Source: CAD feature listing. Evaluate the final solid. Frame: model axes, mm. A direction names the side the tool comes from. Round coordinates to 2 decimals unless told otherwise and drop trailing zeros. Write each loop counter-clockwise with the first axis right and the second up, starting at its lowest first coordinate (ties: lowest second). Pieces come first, ordered by that corner, then holes.
```python
from build123d import *

# Parameters (mm, degrees)
F0_R       = 13.85
F1_DEPTH   = 18.5
F2_R       = 1.5
F3_DEPTH   = 1
F4_R       = 2.5
F5_DEPTH   = 12.5
F6_SIZE2   = 3.4641016151
F6_SIZE    = 2
F6_2_SIZE2 = 3.4641016151
F6_2_SIZE  = 2
F8_D       = 2.5
F8_DEPTH   = 13.5
F8_TIP     = 0.7510757738


with BuildPart() as f1:
    # F0 (on Top) → F1 (new body)
    with BuildSketch(Plane.XY):
        Circle(F0_R)
    extrude(amount=F1_DEPTH)

    # F2 (on face) → F3 (join)
    with BuildSketch(Plane(origin=(0, 0, 0), x_dir=(1, 0, 0), z_dir=(0, 0, -1))):
        Circle(F2_R)
    extrude(amount=F3_DEPTH)

    # F4 (on face) → F5 (join)
    with BuildSketch(Plane.XY.offset(18.5)):
        Circle(F4_R)
    extrude(amount=F5_DEPTH)

    # F6
    f6_edges = [f1.edges().sort_by_distance(p)[0] for p in [
        (-13.85, 0, 18.5),
    ]]
    f6_side = f1.faces().sort_by_distance((-13.458263, 0, 18.5))[0]
    chamfer(f6_edges, length=F6_SIZE, length2=F6_SIZE2, reference=f6_side)

    # F6#2
    f6_2_edges = [f1.edges().sort_by_distance(p)[0] for p in [
        (-13.85, 0, 0),
    ]]
    f6_2_side = f1.faces().sort_by_distance((-13.458263, 0, 0))[0]
    chamfer(f6_2_edges, length=F6_2_SIZE, length2=F6_2_SIZE2, reference=f6_2_side)

    # F8
    with Locations(Plane(origin=(0, 0, 0), x_dir=(1, 0, 0), z_dir=(0, 0, -1))):
        with Locations((-9.5, 0), (0, 8), (9.5, 0), (0, -8)):
            Hole(F8_D / 2, depth=F8_DEPTH)
            with Locations((0, 0, -(F8_DEPTH + F8_TIP / 2))):  # 118° drill point
                Cone(0, F8_D / 2, F8_TIP, mode=Mode.SUBTRACT)


solid = f1.part
```
Q1. Line query: line 1 (Y direction, x = 0.25, z = 3); line 2 (Z direction, x = -2.25, y = -9.25); line 3 (Z direction, x = 0, y = 8). Output: solid intervals per line, ascending.
Q2. Pin query (flat end, axial travel): P1, Ø2, axis at x = 0, y = 8, coming from the +Z side; P2, Ø3, axis at x = 3.5, y = 0, coming from the -Z side; P3, Ø12, axis at x = 5.5, y = -2, coming from the +Z side; P4, Ø5, axis at y = -4.5, z = 25.5, coming from the +X side. Return the tip coordinate at first contact, or that it passes through.
Q3. Set-up query: faces 5 (the face through (-0.54, -2.44, 24.66)), 6 (the face through (-1.5, -0.07, -0.49)), 7 (the face through (13.21, 4.16, 9.17)). Return all of +Z, -Z, +X, -X, +Y, -Y with unobstructed straight access to the full face (end or side cutting, diameter ignored); none if empty.
Q4. Mould query, pull axis Y, two halves, no side actions, for faces 1 (the face through (-8.83, 8.09, 0.22)), 2 (the face through (0, 0, -1)), 3 (the face through (9.7, 0.08, 14.12)), 4 (the face through (0.27, 9.22, 6.84)). Classes: pulls with the +Y half, pulls with the -Y half, needs draft (parallel to the pull), parting line crosses it, or undercut.
Q5. Section query C-C, the plane z = 15.5. Output: boundary loops of the cut face in (x, y).
Q6. Section query B-B, the plane z = 24. Output: boundary loops of the cut face in (x, y), and give its area (3 significant figures).
Q7. Section query A-A, the plane z = 7. Output: boundary loops of the cut face in (x, y), and give its area (3 significant figures).
Filled in:
1. line 1: y = -13.58 to -9.22, -6.78 to 6.78, 9.22 to 13.58
1. line 2: z = 0 to 18.5
1. line 3: z = 14.25 to 18.5
2. P1: stops at z = 18.5
2. P2: stops at z = 0
2. P3: stops at z = 31
2. P4: stops at x = 1.5
3. face 5: +Z
3. face 6: -Z
3. face 7: +Z, -Z
4. face 1: parting line crosses it
4. face 2: needs draft
4. face 3: undercut
4. face 4: undercut
5. outline: circle Ø27.16 at (0, 0)
6. outline: circle Ø5 at (0, 0)
6. area: 19.6 mm2
7. outline: circle Ø27.7 at (0, 0); hole circle Ø2.5 at (-9.5, 0); hole circle Ø2.5 at (0, -8); hole circle Ø2.5 at (0, 8); hole circle Ø2.5 at (9.5, 0)
7. area: 583 mm2
